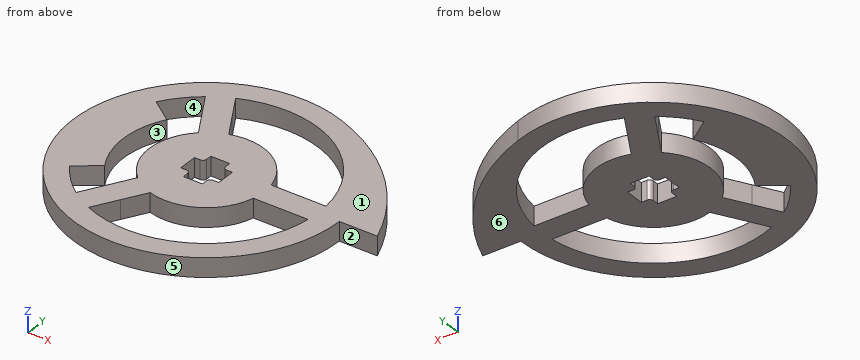
from build123d import *

# Parameters (mm, degrees)
F1_DEPTH = 6.35
F2_R     = 1.27


with BuildPart() as f1:
    # F0 (on Top) → F1 (new body)
    with BuildSketch(Plane.XY):
        with BuildLine():
            ThreePointArc((15.1071694838, 41.7235677075), (-36.3280432516, -25.4824634909), (44.3743470042, 0))
            ThreePointArc((44.3743470042, 0), (36.3280432516, 25.4824634909), (15.1071694838, 41.7235677075))
        make_face()
        with BuildLine():
            ThreePointArc((-14.8868357383, 34.0501787057), (18.5811231374, 32.1834493357), (36.9317376317, 4.1327114215))
            ThreePointArc((36.9317376317, 4.1327114215), (37.1045743636, 2.0695674625), (37.1622462748, 0))
            ThreePointArc((37.1622462748, 0), (37.1045743636, -2.0695674625), (36.9317376317, -4.1327114215))
            ThreePointArc((36.9317376317, -4.1327114215), (18.5811231374, -32.1834493357), (-14.8868357383, -34.0501787057))
            ThreePointArc((-14.8868357383, -34.0501787057), (-18.5811231374, -32.1834493357), (-22.0449018934, -29.9174672842))
            ThreePointArc((-22.0449018934, -29.9174672842), (-27.1515852785, -25.3736864695), (-31.3396552702, -19.9714435065))
            ThreePointArc((-31.3396552702, -19.9714435065), (-37.1622462748, 0), (-31.3396552702, 19.9714435065))
            ThreePointArc((-31.3396552702, 19.9714435065), (-27.1515852785, 25.3736864695), (-22.0449018934, 29.9174672842))
            ThreePointArc((-22.0449018934, 29.9174672842), (-18.5811231374, 32.1834493357), (-14.8868357383, 34.0501787057))
        make_face(mode=Mode.SUBTRACT)
        with BuildLine():
            ThreePointArc((15.1071694838, 41.7235677075), (36.3280432516, 25.4824634909), (44.3743470042, 0))
            Line((44.3743470042, 0), (57.0743470042, 0))
            ThreePointArc((57.0743470042, 0), (40.7796227308, 25.5780250359), (15.1071694838, 41.7235677075))
        make_face()
        with BuildLine():
            ThreePointArc((-9.525, 16.4977839421), (-7.6678534057, 17.4386502961), (-5.7191279813, 18.1712430817))
            Line((-5.7191279813, 18.1712430817), (-10.11946405, 25.792848723))
            ThreePointArc((-10.11946405, 25.792848723), (-13.8534706654, 23.9949150536), (-17.2775302051, 21.6601373015))
            Line((-17.2775302051, 21.6601373015), (-12.8771941364, 14.0385316602))
            ThreePointArc((-12.8771941364, 14.0385316602), (-11.2683874613, 15.3598809898), (-9.525, 16.4977839421))
        make_face()
        with BuildLine():
            ThreePointArc((-17.2775302051, 21.6601373015), (-13.8534706654, 23.9949150536), (-10.11946405, 25.792848723))
            Line((-10.11946405, 25.792848723), (-14.8868357383, 34.0501787057))
            ThreePointArc((-14.8868357383, 34.0501787057), (-18.5811231374, 32.1834493357), (-22.0449018934, 29.9174672842))
            Line((-22.0449018934, 29.9174672842), (-17.2775302051, 21.6601373015))
        make_face()
        with BuildLine():
            Line((-10.11946405, -25.792848723), (-5.7191279813, -18.1712430817))
            ThreePointArc((-5.7191279813, -18.1712430817), (-7.6678534057, -17.4386502961), (-9.525, -16.4977839421))
            ThreePointArc((-9.525, -16.4977839421), (-11.2683874613, -15.3598809898), (-12.8771941364, -14.0385316602))
            Line((-12.8771941364, -14.0385316602), (-17.2775302051, -21.6601373015))
            ThreePointArc((-17.2775302051, -21.6601373015), (-13.8534706654, -23.9949150536), (-10.11946405, -25.792848723))
        make_face()
        with BuildLine():
            Line((-14.8868357383, -34.0501787057), (-10.11946405, -25.792848723))
            ThreePointArc((-10.11946405, -25.792848723), (-13.8534706654, -23.9949150536), (-17.2775302051, -21.6601373015))
            Line((-17.2775302051, -21.6601373015), (-22.0449018934, -29.9174672842))
            ThreePointArc((-22.0449018934, -29.9174672842), (-18.5811231374, -32.1834493357), (-14.8868357383, -34.0501787057))
        make_face()
        with BuildLine():
            ThreePointArc((18.5963221177, 4.1327114215), (18.936240867, 2.0787693062), (19.05, 0))
            ThreePointArc((19.05, 0), (18.936240867, -2.0787693062), (18.5963221177, -4.1327114215))
            Line((18.5963221177, -4.1327114215), (27.3969942551, -4.1327114215))
            ThreePointArc((27.3969942551, -4.1327114215), (27.6293459059, -2.0721589516), (27.7069413308, 0))
            ThreePointArc((27.7069413308, 0), (27.6293459059, 2.0721589516), (27.3969942551, 4.1327114215))
            Line((27.3969942551, 4.1327114215), (18.5963221177, 4.1327114215))
        make_face()
        with BuildLine():
            Line((36.9317376317, 4.1327114215), (27.3969942551, 4.1327114215))
            ThreePointArc((27.3969942551, 4.1327114215), (27.6293459059, 2.0721589516), (27.7069413308, 0))
            ThreePointArc((27.7069413308, 0), (27.6293459059, -2.0721589516), (27.3969942551, -4.1327114215))
            Line((27.3969942551, -4.1327114215), (36.9317376317, -4.1327114215))
            ThreePointArc((36.9317376317, -4.1327114215), (37.1045743636, -2.0695674625), (37.1622462748, 0))
            ThreePointArc((37.1622462748, 0), (37.1045743636, 2.0695674625), (36.9317376317, 4.1327114215))
        make_face()
        with BuildLine():
            ThreePointArc((18.5963221177, -4.1327114215), (18.936240867, -2.0787693062), (19.05, 0))
            ThreePointArc((19.05, 0), (18.936240867, 2.0787693062), (18.5963221177, 4.1327114215))
            ThreePointArc((18.5963221177, 4.1327114215), (9.525, 16.4977839421), (-5.7191279813, 18.1712430817))
            ThreePointArc((-5.7191279813, 18.1712430817), (-7.6678534057, 17.4386502961), (-9.525, 16.4977839421))
            ThreePointArc((-9.525, 16.4977839421), (-11.2683874613, 15.3598809898), (-12.8771941364, 14.0385316602))
            ThreePointArc((-12.8771941364, 14.0385316602), (-19.05, 0), (-12.8771941364, -14.0385316602))
            ThreePointArc((-12.8771941364, -14.0385316602), (-11.2683874613, -15.3598809898), (-9.525, -16.4977839421))
            ThreePointArc((-9.525, -16.4977839421), (-7.6678534057, -17.4386502961), (-5.7191279813, -18.1712430817))
            ThreePointArc((-5.7191279813, -18.1712430817), (9.525, -16.4977839421), (18.5963221177, -4.1327114215))
        make_face()
        Polygon((-3.175, 6.35), (3.175, 6.35), (3.175, 3.175), (6.35, 3.175), (6.35, -3.175), (3.175, -3.175), (3.175, -6.35), (-3.175, -6.35), (-3.175, -3.175), (-6.35, -3.175), (-6.35, 3.175), (-3.175, 3.175), align=None, mode=Mode.SUBTRACT)
        with BuildLine():
            ThreePointArc((-23.6801005032, -14.3849726474), (-27.7069413308, 0), (-23.6801005032, 14.3849726474))
            Line((-23.6801005032, 14.3849726474), (-31.3396552702, 19.9714435065))
            ThreePointArc((-31.3396552702, 19.9714435065), (-37.1622462748, 0), (-31.3396552702, -19.9714435065))
            Line((-31.3396552702, -19.9714435065), (-23.6801005032, -14.3849726474))
        make_face()
    extrude(amount=F1_DEPTH)

    # F2
    f2_edges = [f1.edges().sort_by_distance(p)[0] for p in [
        (-3.175, 3.175, 3.175),
        (-3.175, -3.175, 3.175),
        (3.175, -3.175, 3.175),
        (3.175, 3.175, 3.175),
    ]]
    fillet(f2_edges, radius=F2_R)


solid = f1.part
Check sheet for the modelled part. Datum: model origin and axes. Units: mm. Face numbers are marked on the shaded views. A direction names the side the tool comes from. Coordinates: 2 decimals unless noted, no trailing zeros. Write each loop counter-clockwise with the first axis right and the second up, starting at its lowest first coordinate (ties: lowest second). Pieces come first, ordered by that corner, then holes.
Item 1: Cross-section at B-B on y = -16.5. Record the boundary of the cut face in (x, z), then the cut area to 3 significant figures.
Numbers:
outline: (-41.19, 0) - (-26.58, 0) - (-26.58, 6.35) - (-41.19, 6.35) - close; (-14.3, 0) - (9.52, 0) - (9.52, 6.35) - (-14.3, 6.35) - close; (33.3, 0) - (41.19, 0) - (41.19, 6.35) - (33.3, 6.35) - close
area: 294 mm2
Item 2: Mould release check, pull along X, two halves, no side actions. Record for the marked faces 4, 5 and 6: released by +X, released by -X, zero draft, split by the parting line, or undercut.
Numbers:
face 4: undercut
face 5: split by the parting line
face 6: zero draft
Item 3: Scan lines: probe 1 along X at (y, z) = (1, 5.25); probe 2 along X at (y, z) = (24, 3.5); probe 3 along X at (y, z) = (-5, 5.25) (3 decimals). Record each from-to range of solid material in increasing order.
Numbers:
probe 1: x = -44.36 to -27.69, -19.02 to -6.35, 6.35 to 56.7
probe 2: x = -37.32 to -28.37, -18.63 to -9.08, 28.37 to 42.32
probe 3: x = -44.092 to -27.252, -18.382 to -3.175, 3.175 to 18.382, 36.824 to 44.092
Item 4: Cross-section at A-A on x = 0. Record the boundary of the cut face in (y, z).
Numbers:
outline: (-44.37, 0) - (-37.16, 0) - (-37.16, 6.35) - (-44.37, 6.35) - close; (-19.05, 0) - (-6.35, 0) - (-6.35, 6.35) - (-19.05, 6.35) - close; (6.35, 0) - (19.05, 0) - (19.05, 6.35) - (6.35, 6.35) - close; (37.16, 0) - (44.37, 0) - (44.37, 6.35) - (37.16, 6.35) - close
Item 5: Depth check by flat-ended pin: pin 1 Ø2 at (y, z) = (-34, 5.5) entering from +X; pin 2 Ø6 at (x, y) = (37, -33) entering from -Z; pin 3 Ø2 at (x, z) = (-5.5, 4) entering from -Y; pin 4 Ø1.5 at (y, z) = (-6, 2.5) entering from +X. Enter the tip coordinate at first touch or a pass-through.
Numbers:
pin 1: stops at x = 29.67
pin 2: passes through
pin 3: stops at y = -44.15
pin 4: stops at x = 44.06
Item 6: Cross-section at C-C on x = 34.5. Record the boundary of the cut face in (y, z), then the cut area to 3 significant figures.
Numbers:
outline: (-27.91, 0) - (-13.81, 0) - (-13.81, 6.35) - (-27.91, 6.35) - close; (-4.13, 0) - (4.13, 0) - (4.13, 6.35) - (-4.13, 6.35) - close; (13.81, 0) - (31.11, 0) - (31.11, 6.35) - (13.81, 6.35) - close
area: 252 mm2
Item 7: Access from +Z, -Z, +X, -X, +Y, -Y to the whole of each face (thin tool, end or side, straight path). Record for the marked faces 1, 2 and 3.
Numbers:
face 1: +Z, +X, -X, +Y, -Y
face 2: +Z, -Z, +X, -Y
face 3: +Z, -Z
Item 8: Cross-section at D-D on z = 2.75. Count the separate pieces of the cut face and the enclosed holes in it, then the cut area to 3 significant figures.
Numbers:
separate pieces: 1
enclosed holes: 4
area: 3,910 mm2
